Read the model definition and answer for the solid it produces. Units are mm, in the model's axes. A direction names the side the tool comes from. Give positions to 0.01 mm unless a question says otherwise; leave off trailing zeros. Write each loop counter-clockwise with the first axis right and the second up, starting at its lowest first coordinate (ties: lowest second). Pieces come first, ordered by that corner, then holes. Notation, with made-up numbers: (6.25, -26) -> (26.25, -26) arc R16 cw to (26.25, 4) -> close; hole circle Ø8 at (47, -3). An arc over 180 degrees is marked (long way). Use a Markdown table: item, result.
from build123d import *

# Parameters (mm, degrees)
SKETCH_W     = 42.3
SKETCH_H     = 42.3
PAD_DEPTH    = 38
SKETCH001_R  = 1.7
HOLE_DEPTH   = 4.5
HOLE_TIPS_R  = 1.7
SKETCH002_R  = 11
PAD001_DEPTH = 2
FILLET_R     = 0.5
CHAMFER_SIZE = 3
SKETCH003_R  = 2.5
PAD002_DEPTH = 21.5
POCKET_DEPTH = 18
FILLET001_R  = 0.25
SKETCH005_W  = 16.2
SKETCH005_H  = 9.4
PAD003_DEPTH = 5


with BuildPart() as part:
    # Sketch → Pad (new body)
    with BuildSketch(Plane.XZ):
        Rectangle(SKETCH_W, SKETCH_H)
    extrude(amount=PAD_DEPTH)

    # Sketch001 (on Face6 of Pad) → Hole (cut)
    with BuildSketch(Plane.XZ.offset(38)):
        with Locations((-15.5, 15.5)):
            Circle(SKETCH001_R)
        with Locations((15.5, 15.5)):
            Circle(SKETCH001_R)
        with Locations((15.5, -15.5)):
            Circle(SKETCH001_R)
        with Locations((-15.5, -15.5)):
            Circle(SKETCH001_R)
    extrude(amount=-HOLE_DEPTH, mode=Mode.SUBTRACT)

    # Hole tips → Hole tip 1 section 0
    with BuildSketch(Plane.XZ.offset(33.5), mode=Mode.PRIVATE) as hole_tip_1_s0:
        with Locations((-15.5, 15.5)):
            Circle(HOLE_TIPS_R)
    loft([hole_tip_1_s0.sketch, Vertex(-15.5, -32.478537, 15.5)], mode=Mode.SUBTRACT)

    # Hole tips → Hole tip 2 section 0
    with BuildSketch(Plane.XZ.offset(33.5), mode=Mode.PRIVATE) as hole_tip_2_s0:
        with Locations((15.5, 15.5)):
            Circle(HOLE_TIPS_R)
    loft([hole_tip_2_s0.sketch, Vertex(15.5, -32.478537, 15.5)], mode=Mode.SUBTRACT)

    # Hole tips → Hole tip 3 section 0
    with BuildSketch(Plane.XZ.offset(33.5), mode=Mode.PRIVATE) as hole_tip_3_s0:
        with Locations((15.5, -15.5)):
            Circle(HOLE_TIPS_R)
    loft([hole_tip_3_s0.sketch, Vertex(15.5, -32.478537, -15.5)], mode=Mode.SUBTRACT)

    # Hole tips → Hole tip 4 section 0
    with BuildSketch(Plane.XZ.offset(33.5), mode=Mode.PRIVATE) as hole_tip_4_s0:
        with Locations((-15.5, -15.5)):
            Circle(HOLE_TIPS_R)
    loft([hole_tip_4_s0.sketch, Vertex(-15.5, -32.478537, -15.5)], mode=Mode.SUBTRACT)

    # Sketch002 (on Face5 of Hole) → Pad001 (join)
    with BuildSketch(Plane.XZ.offset(38)):
        Circle(SKETCH002_R)
    extrude(amount=PAD001_DEPTH)

    # Fillet
    fillet_edges = [part.edges().sort_by_distance(p)[0] for p in [
        (-11, -40, 0),
    ]]
    fillet(fillet_edges, radius=FILLET_R)

    # Chamfer
    chamfer_edges = [part.edges().sort_by_distance(p)[0] for p in [
        (-21.15, -19, -21.15),
        (-21.15, -19, 21.15),
        (21.15, -19, 21.15),
        (21.15, -19, -21.15),
    ]]
    chamfer(chamfer_edges, length=CHAMFER_SIZE)

    # Sketch003 (on Face21 of Chamfer) → Pad002 (join)
    with BuildSketch(Plane.XZ.offset(40)):
        Circle(SKETCH003_R)
    extrude(amount=PAD002_DEPTH)

    # Sketch004 (on Face23 of Pad002) → Pocket (cut)
    with BuildSketch(Plane.XZ.offset(61.5)):
        with BuildLine():
            Line((-1.5, 2), (1.5, 2))
            ThreePointArc((1.5, 2), (0, 2.5), (-1.5, 2))
        make_face()
    extrude(amount=-POCKET_DEPTH, mode=Mode.SUBTRACT)

    # Fillet001
    fillet001_edges = [part.edges().sort_by_distance(p)[0] for p in [
        (-1.118034, -61.5, -2.236068),
        (0, -61.5, 2),
        (2.236068, -61.5, 1.118034),
    ]]
    fillet(fillet001_edges, radius=FILLET001_R)

    # Sketch005 (on Face19 of Fillet001) → Pad003 (join)
    with BuildSketch(Plane(origin=(0, 0, 21.15), x_dir=(-1, 0, 0), z_dir=(0, 0, 1))):
        with Locations((0, 4.7)):
            Rectangle(SKETCH005_W, SKETCH005_H)
    extrude(amount=PAD003_DEPTH)


solid = part.part
Item 1: A tool of negligible diameter and unlimited length cuts with its end or side. For faces 4 (the face through (8.1, -5, 24)), 5 (the face through (-0.54, -50.48, -2.44)), 6 (the face through (0, -9.4, 24)), from which of +Z, -Z, +X, -X, +Y, -Y can it reach the whole face along a straight path? Write none if from no direction.
Return value:
| item | result |
|---|---|
| face 4 | +Z, +X, +Y, -Y |
| face 5 | -Y |
| face 6 | +Z, +X, -X, -Y |
Item 2: For a pull along X with two mould halves and no side action, classify faces 1 (the face through (0, 0, 3)), 2 (the face through (21.15, -19, 0)), 3 (the face through (17.07, -35.78, 14.85)) as +X half, -X half, draft (parallel to the pull), parting line (faces both ways), or undercut.
Return value:
| item | result |
|---|---|
| face 1 | draft |
| face 2 | +X half |
| face 3 | undercut |
Item 3: A cutting plane is placed at C-C (y = -57.5). Give the vertices of the cut face in (x, z), then the cut area to 3 significant figures.
Return value:
| item | result |
|---|---|
| outline | (-1.5, 2) arc R2.5 ccw (long way) to (1.5, 2) -> close |
| area | 18.6 mm^2 |
Item 4: Straight lines are drawn through the part: line 1 along Z through (x, y) = (-15.5, -35.55); line 2 along Z through (x, y) = (-17, -34.5); line 3 along X through (y, z) = (-35, -15). For each, find the intervals that lie inside material, in ascending order. Write a range as [from, to].
Return value:
| item | result |
|---|---|
| line 1 | [-21.15, -17.2], [-13.8, 13.8], [17.2, 21.15] |
| line 2 | [-21.15, -16.3], [-14.7, 14.7], [16.3, 21.15] |
| line 3 | [-21.15, -17.12], [-13.88, 13.88], [17.12, 21.15] |
Item 5: A cutting plane is placed at B-B (z = 12.5). Give the vertices of the cut face in (x, y), then the cut area to 3 significant figures.
Return value:
| item | result |
|---|---|
| outline | (-21.15, -38) -> (21.15, -38) -> (21.15, 0) -> (-21.15, 0) -> close |
| area | 1,610 mm^2 |
Item 6: A cutting plane is placed at A-A (y = -16). Give the vertices of the cut face in (x, z), then the cut area to 3 significant figures.
Return value:
| item | result |
|---|---|
| outline | (-21.15, -18.15) -> (-18.15, -21.15) -> (18.15, -21.15) -> (21.15, -18.15) -> (21.15, 18.15) -> (18.15, 21.15) -> (-18.15, 21.15) -> (-21.15, 18.15) -> close |
| area | 1,770 mm^2 |
Item 7: Each of these flat-tipped pins is pushed along its axis until it touches: P1, Ø4.5, axis at x = -15.5, z = -15.5, coming from the -Y side; P2, Ø5.5, axis at y = -5.5, z = 23.5, coming from the +X side; P3, Ø2.5, axis at x = 1, z = 23, coming from the -Y side. Where does it stop, or does it pass through?
Return value:
| item | result |
|---|---|
| P1 | y = -38 |
| P2 | x = 18.55 |
| P3 | y = -9.4 |
